For this review, take the finished solid that the model builds, in its own axes (mm). Give positions to 0.01 mm unless a question says otherwise; leave off trailing zeros. Order: outer loops, then holes, each group sorted by start corner. A loop starts at its lowest first (then second) coordinate and runs counter-clockwise, first axis right, second up. Notation, with made-up numbers: (50.25, 19) -> (93.25, 19) arc R27 ccw to (93.25, 43) -> close; hole circle Ø10 at (44, 28.5). An arc over 180 degrees is marked (long way). One line per item, written item: value. Start each with the question number.
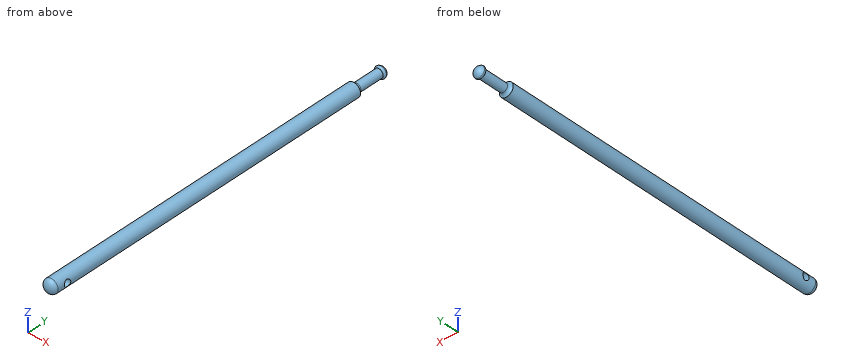
from build123d import *

# Parameters (mm, degrees)
SKETCH1_R               = 2
BOSS_EXTRUDE1_DEPTH     = 104
DOME2_FACE_RADIUS       = 2
DOME2_HEIGHT            = 1.5
CUT_EXTRUDE1_DEPTH      = 105.038454433
CUT_EXTRUDE1_DEPTH_BACK = 105.038454433
SKETCH2_R               = 1
SKETCH6_W               = 0.75
SKETCH6_H               = 8
FILLET1_R               = 0.5
FILLET2_R               = 1


with BuildPart() as part:
    # Sketch1 → Boss-Extrude1 (new body)
    with BuildSketch(Plane(origin=(0, 0, 0), x_dir=(1, 0, 0), z_dir=(0, 1, 0))):
        with Locations(Location((0, 0, 0), (0, 0, 90))):
            Circle(SKETCH1_R)
    extrude(amount=BOSS_EXTRUDE1_DEPTH)

    # Dome2: an elliptical dome of height H over a round flat face of radius A is half a spheroid: the quarter ellipse of half axes A and H revolved about the face's axis
    with BuildSketch(Plane((0, 0, 0), x_dir=(0, 0, 1), z_dir=(1, 0, 0)), mode=Mode.PRIVATE) as dome2_quarter:
        Ellipse(DOME2_FACE_RADIUS, DOME2_HEIGHT)
        Rectangle(DOME2_FACE_RADIUS, DOME2_HEIGHT, align=(Align.MIN, Align.MIN), mode=Mode.INTERSECT)
    revolve(dome2_quarter.sketch, axis=Axis((0, 0, 0), (0, -1, 0)))

    # Sketch2 → Cut-Extrude1 (cut, two sides: drawn at the far end of the back side and taken through both)
    with BuildSketch(Plane(origin=(0, 0, 0), x_dir=(0, 0, -1), z_dir=(1, 0, 0)).offset(-CUT_EXTRUDE1_DEPTH_BACK)):
        with Locations((0, 3)):
            Circle(SKETCH2_R)
    extrude(amount=CUT_EXTRUDE1_DEPTH + CUT_EXTRUDE1_DEPTH_BACK, mode=Mode.SUBTRACT)

    # Sketch5 → Revolve1 (revolve)
    with BuildSketch(Plane.XY):
        with BuildLine():
            Line((0, 102.25), (0, 105.75))
            ThreePointArc((0, 105.75), (1.75, 104), (0, 102.25))
        make_face()
    revolve(axis=Axis((0, 102.25, 0), (0, 1, 0)))

    # Sketch6 → Cut-Revolve1 (revolve, cut)
    with BuildSketch(Plane.XY, mode=Mode.PRIVATE) as cut_revolve1_sk:
        with Locations((1.625, 100)):
            Rectangle(SKETCH6_W, SKETCH6_H)
    revolve(cut_revolve1_sk.sketch.rotate(Axis((0, 105.75, 0), (0, -1, 0)), 180), axis=Axis((0, 105.75, 0), (0, -1, 0)), mode=Mode.SUBTRACT)

    # Fillet1
    # the kernel refuses this fillet: 0.5 mm, written as the material it takes off along each edge
    with BuildSketch(Plane(origin=(0, 104, 0), x_dir=(1, 0, 0), z_dir=(0, 0, -1))) as fillet1_piece_1:
        with BuildLine():
            CenterArc((1.15, -0.489897949), FILLET1_R, 336.926081934, 101.536959033)
            Line((1.61, -0.685857128), (1.6192, -0.689776312))
            ThreePointArc((1.6192, -0.689776312), (1.724440779, -0.352), (1.76, 0))
            Line((1.76, 0), (1.75, 0.01))
            ThreePointArc((1.75, 0.01), (1.5, 0.01), (1.252, 0.009797959))
            Line((1.252, 0.009797959), (1.25, 0))
        make_face()
    revolve(axis=Axis((0, 104, 0), (0, -1, 0)), mode=Mode.SUBTRACT)

    # Fillet2
    # the kernel refuses this fillet: 1 mm, written as the material it adds along each edge
    with BuildSketch(Plane(origin=(0, 96, 0), x_dir=(-1, 0, 0), z_dir=(0, 0, 1))) as fillet2_piece_1:
        with BuildLine():
            CenterArc((2.25, -0.968245837), FILLET2_R, 104.477512186, 75.522487814)
            Line((1.25, -0.968245837), (1.23, -0.968245837))
            Line((1.23, -0.968245837), (1.23, 0))
            Line((1.23, 0), (1.25, 0.02))
            ThreePointArc((1.25, 0.02), (1.625, 0.02), (1.995, 0.019364917))
            Line((1.995, 0.019364917), (2, 0))
        make_face()
    revolve(axis=Axis((0, 96, 0), (0, -1, 0)))


solid = part.part
Q1. For pin 1 Ø2 at (x, z) = (1.5, 1) entering from -Y; pin 2 Ø1.8 at (y, z) = (3, 0) entering from -X; pin 3 Ø1.5 at (x, z) = (-1, -1.5) entering from -Y; pin 4 Ø1 at (x, z) = (-0.5, -0.5) entering from +Y, all flat-tipped, find the tip position at first contact; note any pin that passes through.
Q2. For line 1 along Z through (x, y) = (-0.05, 3); line 2 along Y through (x, z) = (-1.5, 0.2); line 3 along X through (y, z) = (39, 0.25), list the stretches that pass through material, from the lowest coordinate up.
Q3. Take a section at A-A (y = 86.5). State the section outline as (x, z) points.
Q4. Take a section at B-B (y = 3). State the section outline as (x, z) points, and give its area (3 significant figures).
Answers below:
1. pin 1: stops at y = -1.37
1. pin 2: passes through
1. pin 3: stops at y = -1.28
1. pin 4: stops at y = 105.74
2. line 1: z = -2 to -1, 1 to 2
2. line 2: y = -0.98 to 2.02, 3.98 to 96.29, 104.15 to 104.88
2. line 3: x = -1.98 to 1.98
3. outline: circle Ø4 at (0, 0)
4. outline: (-1.73, -1) arc R2 ccw to (1.73, -1) -> close; (-1.73, 1) -> (1.73, 1) arc R2 ccw to start
4. area: 4.91 mm²
